Source: CAD feature listing. Evaluate the final solid. Frame: model axes, mm. Face numbers are marked on the shaded views. Give positions to 0.01 mm unless a question says otherwise; leave off trailing zeros. Order: outer loops, then holes, each group sorted by start corner. A loop starts at its lowest first (then second) coordinate and runs counter-clockwise, first axis right, second up. Notation, with made-up numbers: (74, -28) -> (133, -28) arc R33 cw to (133, 9) -> close; hole circle Ø11 at (67, -36.75). An arc over 180 degrees is marked (long way). Use CSV: the item, a comma, the result in double quotes.
```python
from build123d import *

# Parameters (mm, degrees)
SKETCH1_W                        = 77.3
SKETCH1_H                        = 57.3
BOSS_EXTRUDE1_DEPTH              = 6
SKETCH2_R                        = 8
SKETCH2_R_2                      = 2.6
CUT_EXTRUDE1_DEPTH               = 6
TAP_DRILL_FOR_M6_HELICOIL1_D     = 6.25
TAP_DRILL_FOR_M6_HELICOIL1_DEPTH = 20
TAP_DRILL_FOR_M6_HELICOIL1_TIP   = 1.877689434


with BuildPart() as part:
    # Sketch1 → Boss-Extrude1 (new body)
    with BuildSketch(Plane.XY):
        Rectangle(SKETCH1_W, SKETCH1_H)
    extrude(amount=BOSS_EXTRUDE1_DEPTH)

    # Sketch2 → Cut-Extrude1 (cut)
    with BuildSketch(Plane.XY.offset(6)):
        with Locations((10, 0)):
            Circle(SKETCH2_R)
        with Locations((-13.57, 23.57)):
            Circle(SKETCH2_R_2)
        with Locations((33.57, 23.57)):
            Circle(SKETCH2_R_2)
        with Locations((33.57, -23.57)):
            Circle(SKETCH2_R_2)
        with Locations((-13.57, -23.57)):
            Circle(SKETCH2_R_2)
    extrude(amount=-CUT_EXTRUDE1_DEPTH, mode=Mode.SUBTRACT)

    # Tap Drill for M6 Helicoil1
    with Locations(Plane(origin=(-28.65, 14.325, 6), x_dir=(1, 0, 0), z_dir=(0, 0, 1))):
        with Locations((0, 0), (0, -28.65)):
            Hole(TAP_DRILL_FOR_M6_HELICOIL1_D / 2, depth=TAP_DRILL_FOR_M6_HELICOIL1_DEPTH)
            with Locations((0, 0, -(TAP_DRILL_FOR_M6_HELICOIL1_DEPTH + TAP_DRILL_FOR_M6_HELICOIL1_TIP / 2))):  # 118° drill point
                Cone(0, TAP_DRILL_FOR_M6_HELICOIL1_D / 2, TAP_DRILL_FOR_M6_HELICOIL1_TIP, mode=Mode.SUBTRACT)


solid = part.part
```
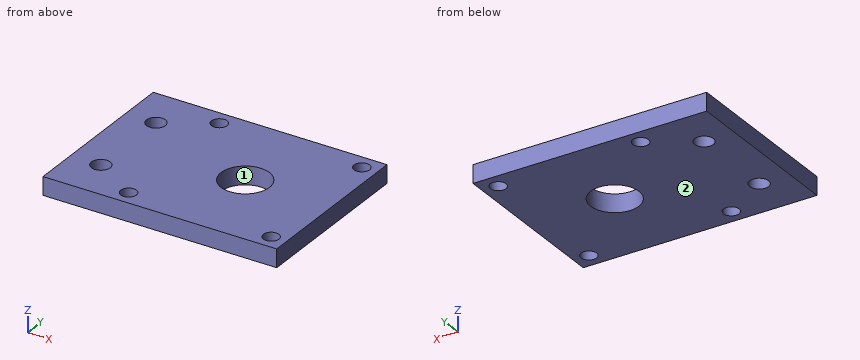
1. Section query C-C on y = 3.5. Return loops of the section in (x, z).
Answer below:
outline,"(-38.65, 0) -> (2.81, 0) -> (2.81, 6) -> (-38.65, 6) -> close; (17.19, 0) -> (38.65, 0) -> (38.65, 6) -> (17.19, 6) -> close"
2. Section query D-D on z = 1.7. Return loops of the section in (x, y) (3 decimals).
Answer below:
outline,"(-38.65, -28.65) -> (38.65, -28.65) -> (38.65, 28.65) -> (-38.65, 28.65) -> close; hole circle Ø6.25 at (-28.65, -14.325); hole circle Ø6.25 at (-28.65, 14.325); hole circle Ø5.2 at (-13.57, -23.57); hole circle Ø5.2 at (-13.57, 23.57); hole circle Ø16 at (10, 0); hole circle Ø5.2 at (33.57, -23.57); hole circle Ø5.2 at (33.57, 23.57)"
3. Section query B-B on y = 23.57. Return loops of the section in (x, z), plus the area to 3 significant figures.
Answer below:
outline,"(-38.65, 0) -> (-16.17, 0) -> (-16.17, 6) -> (-38.65, 6) -> close; (-10.97, 0) -> (30.97, 0) -> (30.97, 6) -> (-10.97, 6) -> close; (36.17, 0) -> (38.65, 0) -> (38.65, 6) -> (36.17, 6) -> close"
area,"401 mm²"
4. Mould query, pull axis X, two halves, no side actions, for the marked faces 1 and 2. Classes: released by +X, released by -X, zero draft, split by the parting line, or undercut.
Answer below:
face 1,"undercut"
face 2,"zero draft"
5. Section query A-A on x = -28.65. Return loops of the section in (y, z), plus the area to 3 significant figures.
Answer below:
outline,"(-28.65, 0) -> (-17.45, 0) -> (-17.45, 6) -> (-28.65, 6) -> close; (-11.2, 0) -> (11.2, 0) -> (11.2, 6) -> (-11.2, 6) -> close; (17.45, 0) -> (28.65, 0) -> (28.65, 6) -> (17.45, 6) -> close"
area,"269 mm²"
6. Ray query, line 1 along Y through (x, z) = (-28.65, 2.05); line 2 along Y through (x, z) = (33.57, 1.75); line 3 along X through (y, z) = (0.5, 0.9). Return the intervals inside material, ascending.
Answer below:
line 1,"y = -28.65 to -17.45, -11.2 to 11.2, 17.45 to 28.65"
line 2,"y = -28.65 to -26.17, -20.97 to 20.97, 26.17 to 28.65"
line 3,"x = -38.65 to 2.02, 17.98 to 38.65"
